Work out the finished part from the listing and answer in its coordinate system (mm). Give positions to 0.01 mm unless a question says otherwise; leave off trailing zeros. Order: outer loops, then holes, each group sorted by start corner. A loop starts at its lowest first (then second) coordinate and runs counter-clockwise, first axis right, second up. Notation, with made-up numbers: M 45,2 L 79,2 A25 ccw 79,16 Z; hole C 26,22.5 d6. An arc over 180 degrees is marked long. One line per item, written item: value.
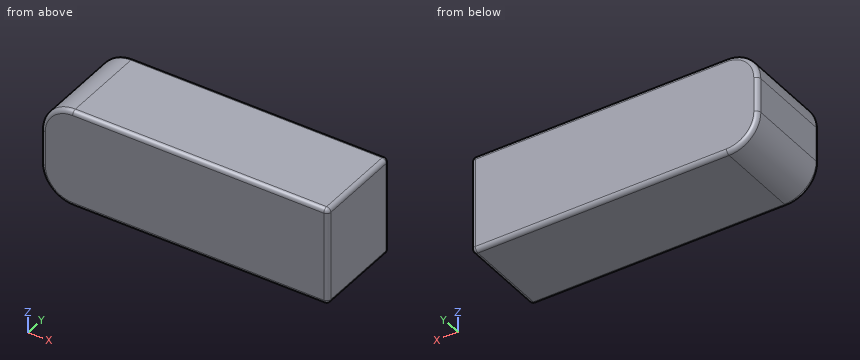
from build123d import *

# Parameters (mm, degrees)
SKETCH1_W           = 136
SKETCH1_H           = 46.4
BOSS_EXTRUDE1_DEPTH = 43.5
FILLET1_R           = 15
FILLET2_R           = 2


with BuildPart() as part:
    # Sketch1 → Boss-Extrude1 (new body)
    with BuildSketch(Plane(origin=(0, 0, 0), x_dir=(1, 0, 0), z_dir=(0, 1, 0))):
        Rectangle(SKETCH1_W, SKETCH1_H)
    extrude(amount=BOSS_EXTRUDE1_DEPTH)

    # Fillet1
    fillet1_edges = [part.edges().sort_by_distance(p)[0] for p in [
        (-68, 21.75, 23.2),
        (-68, 21.75, -23.2),
    ]]
    fillet(fillet1_edges, radius=FILLET1_R)

    # Fillet2
    fillet2_edges = [part.edges().sort_by_distance(p)[0] for p in [
        (-68, 0, 0),
        (-68, 43.5, 0),
        (7.5, 0, 23.2),
        (-63.606601718, 0, 18.806601718),
        (-63.606601718, 0, -18.806601718),
        (7.5, 43.5, 23.2),
        (-63.606601718, 43.5, 18.806601718),
        (-63.606601718, 43.5, -18.806601718),
        (68, 43.5, 0),
        (7.5, 0, -23.2),
        (68, 0, 0),
        (7.5, 43.5, -23.2),
        (68, 21.75, 23.2),
        (68, 21.75, -23.2),
    ]]
    fillet(fillet2_edges, radius=FILLET2_R)


solid = part.part
(1) Section A-A, the plane y = 12 is taken. Give the vertices of the cut face in (x, z).
Findings:
outline: M -68,-8.2 A15 ccw -53,-23.2 L 66,-23.2 A2 ccw 68,-21.2 L 68,21.2 A2 ccw 66,23.2 L -53,23.2 A15 ccw -68,8.2 Z
(2) Given P1, Ø10, axis at y = 12.5, z = -10, coming from the -X side; P2, Ø5, axis at y = 14, z = 14, coming from the -X side, each flat-ended and moving along its own axis, determine where each tip first touches the part or whether it passes through.
Findings:
P1: stops at x = -68
P2: stops at x = -67.63
(3) Find the intervals of material crossed by probe 1 along X at (y, z) = (15, -16.5); probe 2 along X at (y, z) = (24, -15); probe 3 along Z at (x, y) = (-55, 24), in increasing order. Write a range as from..to.
Findings:
probe 1: x = -65.49..68
probe 2: x = -66.37..68
probe 3: z = -23.07..23.07
